Here's the drawing with two shaded views (mm, measured from the low corner). I have some questions. Give positions to 0.01 mm unless a question says otherwise; leave off trailing zeros. Loops run counter-clockwise (first coordinate to the right, second up) from the corner with the lowest first, then second, coordinate; pieces in that order, holes last. Notation, with made-up numbers: (69.5, 64) -> (128.5, 64) arc R24 ccw to (128.5, 84) -> close; hole circle Ø3 at (20, -35). An arc over 180 degrees is marked (long way). Answer in a Markdown table with one row per item. Add a question column.
Item 1: If I drill on line 1 (X direction, y = 21.5, z = 1.45); line 2 (X direction, y = 7.5, z = 2.1); line 3 (Y direction, x = 29.5, z = 1.25), over which ranges is the centre line in solid material (lowest first)?
Item 2: If we section it at C-C (z = 1): Write out the boundary of the cut face in (x, y).
Item 3: If we section it at A-A (y = 9.75): Write out the boundary of the cut face in (x, z), then the cut area to 3 significant figures.
Item 4: If we section it at B-B (x = 8): Write out the boundary of the cut face in (y, z).
Item 5: We'd pull the mould along Y, two halves only. Please class the marked faces 1, 2 and 3: released by +Y, released by -Y, zero draft, split by the parting line, or undercut.
Item 6: If we section it at D-D (x = 43): Write out the boundary of the cut face in (y, z), then the cut area to 3 significant figures.
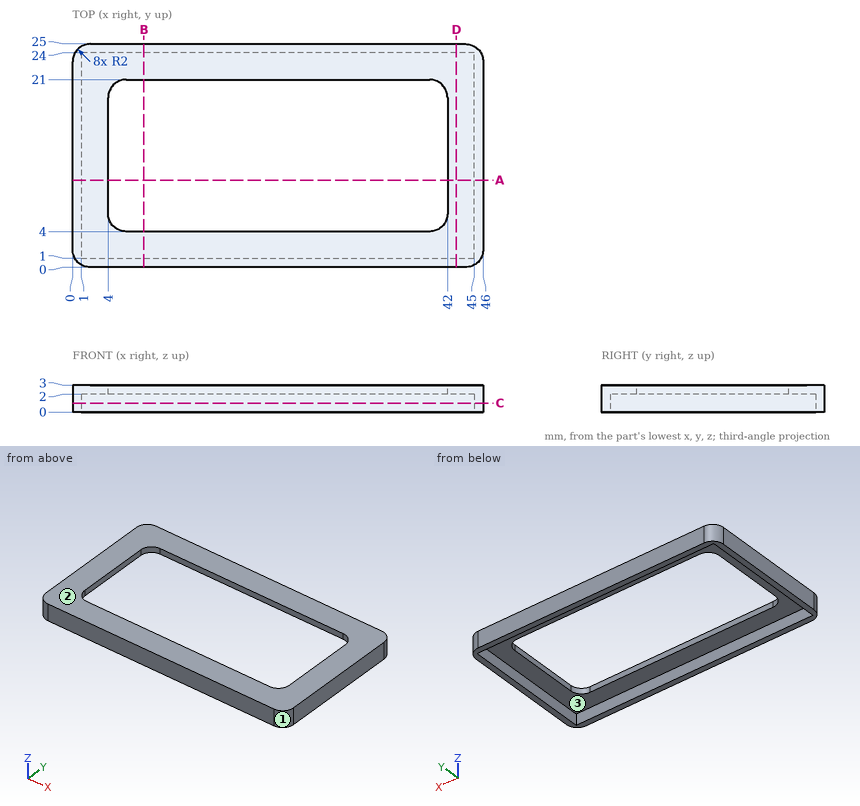
Recorded:
| question | item | result |
|---|---|---|
| 1 | line 1 | x = 0 to 1, 45 to 46 |
| 1 | line 2 | x = 0 to 4, 42 to 46 |
| 1 | line 3 | y = 0 to 1, 24 to 25 |
| 2 | outline | (0, 2) arc R2 ccw to (2, 0) -> (44, 0) arc R2 ccw to (46, 2) -> (46, 23) arc R2 ccw to (44, 25) -> (2, 25) arc R2 ccw to (0, 23) -> close; hole (1, 1) -> (45, 1) -> (45, 24) -> (1, 24) -> close |
| 3 | outline | (0, 0) -> (1, 0) -> (1, 2) -> (4, 2) -> (4, 3) -> (0, 3) -> close; (42, 2) -> (45, 2) -> (45, 0) -> (46, 0) -> (46, 3) -> (42, 3) -> close |
| 3 | area | 12.0 mm^2 |
| 4 | outline | (0, 0) -> (1, 0) -> (1, 2) -> (4, 2) -> (4, 3) -> (0, 3) -> close; (21, 2) -> (24, 2) -> (24, 0) -> (25, 0) -> (25, 3) -> (21, 3) -> close |
| 5 | face 1 | released by -Y |
| 5 | face 2 | zero draft |
| 5 | face 3 | undercut |
| 6 | outline | (0, 0) -> (1, 0) -> (1, 2) -> (24, 2) -> (24, 0) -> (25, 0) -> (25, 3) -> (0, 3) -> close |
| 6 | area | 29.0 mm^2 |
